Input: part model. Units: mm. Frame: model coordinates. A direction names the side the tool comes from. Round coordinates to 2 decimals unless told otherwise and drop trailing zeros. Write each loop counter-clockwise with the first axis right and the second up, starting at its lowest first coordinate (ties: lowest second). Pieces come first, ordered by that corner, then holes. Notation, with made-up numbers: M -33,3.5 L 3,3.5 A21 ccw 3,9.5 Z; hole C -32.75,30.25 d1. An arc over 180 degrees is marked long. Write each question's results on one line, items separated by ' | '. Start each with the question number.
```python
from build123d import *

# Parameters (mm, degrees)
REVOLVE1_ANGLE           = 72
REVOLVE1_OTHER_WAY_ANGLE = 8
CUT_EXTRUDE2_DEPTH       = 127.694588784
CUT_EXTRUDE2_DEPTH_BACK  = 127.694588784
SKETCH5_R                = 2.5
CUT_EXTRUDE3_DEPTH       = 127.694588784
CIRPATTERN1_COUNT        = 2
CIRPATTERN1_ANGLE        = 72


with BuildPart() as part:
    # Sketch1 → Revolve1 (revolve)
    with BuildSketch(Plane.XY):
        Polygon((75, 25), (75, 12.5), (70, 7.5), (70, -7.5), (75, -12.5), (75, -25), (80, -25), (90, -15), (90, 15), (80, 25), align=None)
    revolve(axis=Axis((0, 54.030986193, 0), (0, -1, 0)), revolution_arc=REVOLVE1_ANGLE)

    # Sketch1 → Revolve1 other way (revolve)
    with BuildSketch(Plane.XY):
        Polygon((75, 25), (75, 12.5), (70, 7.5), (70, -7.5), (75, -12.5), (75, -25), (80, -25), (90, -15), (90, 15), (80, 25), align=None)
    revolve(axis=Axis((0, 54.030986193, 0), (0, 1, 0)), revolution_arc=REVOLVE1_OTHER_WAY_ANGLE)

    # Sketch2 → Cut-Extrude2 (cut, two sides: drawn at the far end of the back side and taken through both)
    with BuildSketch(Plane(origin=(0, 0, 0), x_dir=(1, 0, 0), z_dir=(0, 1, 0)).offset(-CUT_EXTRUDE2_DEPTH_BACK)):
        with BuildLine():
            ThreePointArc((76.745775327, 10.785915324), (77.311213895, 5.406126715), (77.5, 0))
            Line((77.5, 0), (90, 0))
            ThreePointArc((90, 0), (89.780764523, 6.278082637), (89.124126187, 12.525579086))
            Line((89.124126187, 12.525579086), (76.745775327, 10.785915324))
        make_face()
        with BuildLine():
            Line((33.973763876, -69.656538588), (30.685980275, -62.915583241))
            ThreePointArc((30.685980275, -62.915583241), (26.222461539, -64.90286982), (21.631189606, -66.573956141))
            Line((21.631189606, -66.573956141), (23.176274578, -71.329238722))
            Line((23.176274578, -71.329238722), (23.948817064, -73.706880013))
            ThreePointArc((23.948817064, -73.706880013), (29.03201099, -71.856748729), (33.973763876, -69.656538588))
        make_face()
    extrude(amount=CUT_EXTRUDE2_DEPTH + CUT_EXTRUDE2_DEPTH_BACK, mode=Mode.SUBTRACT)

    # Sketch5 → Cut-Extrude3 (cut, through all)
    with BuildSketch(Plane(origin=(0, 0, 0), x_dir=(0.9271838545667883, 0, -0.3746065934159098), z_dir=(0.3746065934159098, 0, 0.9271838545667883))):
        with Locations(Location((0, 0, 0), (0, 0, 180))):
            Circle(SKETCH5_R)
    cut_extrude3 = extrude(amount=CUT_EXTRUDE3_DEPTH, mode=Mode.SUBTRACT)

    # CirPattern1: Cut-Extrude3 ×2 about axis
    cirpattern1_axis = Axis((0, 54.030986193, 0), (0, 1, 0))
    for i in range(1, CIRPATTERN1_COUNT):
        add(cut_extrude3.rotate(cirpattern1_axis, i * CIRPATTERN1_ANGLE / (CIRPATTERN1_COUNT - 1)), mode=Mode.SUBTRACT)


solid = part.part
```
1. Cut plane B-B on y = -22. Output: boundary loops of the cut face in (x, z).
2. Access query for faces 5 (the face through (25.586, -0.35, 73.155)), 6 (the face through (65.91, 18.66, 35.79)), 7 (the face through (33.04, -1.69, 76.86)), 8 (the face through (84, 0, 0)). Directions: +Z, -Z, +X, -X, +Y, -Y. A direction counts if a zero-diameter tool reaches every point of the face in a straight line with its end or side. Return the directions, or none.
3. Line query: L1, parallel to Z at x = 73, y = -2; L2, parallel to Z at x = 68, y = 22; L3, parallel to X at y = -7, z = 56. Output: solid intervals per line, ascending. Write a range as from..to.
4. Cut plane A-A on y = 4. Output: boundary loops of the cut face in (x, z).
5. Contact query for flat-ended pins moving along their axis: P1, Ø1, axis at x = 37, y = -16.5, coming from the -Z side; P2, Ø10, axis at x = 34.5, y = -5, coming from the +Z side; P3, Ø1, axis at x = 32.5, y = -9.5, coming from the -Z side. Output: stop coordinate, or through.
6. Draft query along Z for faces 1 (the face through (65, -25, 39)), 2 (the face through (73.36, 1.52, -7.12)), 3 (the face through (66.482, 22.292, 49.201)), 4 (the face through (65.91, -18.84, 35.79)). Return one class per face: +Z half, -Z half, draft (parallel to the pull), parting line (faces both ways), or undercut.
Answers follow:
1) outline: M 23.95,73.71 A77.5 cw 33.97,69.66 L 32.88,67.41 A75 cw 74.27,-10.44 L 76.75,-10.79 A77.5 ccw 77.5,0 L 83,0 A83 ccw 25.65,78.94 Z
2) face 5: -X, +Y, -Y | face 6: -X, +Y | face 7: none | face 8: -Z, +X, +Y, -Y
3) L1: z = -10.26..-6.61, -3.6..52.64 | L2: z = 31.64..47.59 | L3: x = 42..70.46
4) outline: M 23.95,73.71 A77.5 cw 33.97,69.66 L 30.69,62.92 A70 cw 69.32,-9.74 L 76.75,-10.79 A77.5 ccw 77.5,0 L 90,0 A90 ccw 27.81,85.6 Z
5) P1: stops at z = 64.95 | P2: stops at z = 85.03 | P3: stops at z = 63.63
6) face 1: draft | face 2: undercut | face 3: +Z half | face 4: undercut
